Model file for the job. Use its own axes, mm. Face numbers are marked on the shaded views. A direction names the side the tool comes from. Round coordinates to 2 decimals unless told otherwise and drop trailing zeros. Order: outer loops, then holes, each group sorted by start corner. A loop starts at its lowest first (then second) coordinate and runs counter-clockwise, first axis right, second up. Notation, with made-up numbers: (85, 19.5) - (124, 19.5) arc R24 cw to (124, 45.5) - close; hole circle Ø10 at (49.5, 61.25). An arc over 180 degrees is marked (long way). Answer as CSV lines item,"result". Start each with the question number.
1. Band-saw the part on B-B on z = 21.75. List the corners of the cut face in (x, y) (3 decimals).
2. Wall check: line 1 along Y through (x, z) = (0, 26.65); line 2 along X through (y, z) = (13.5, 34); line 3 along Y through (x, z) = (20, 31.75). Give the ranges that are in metal, low to high. Write a range as [from, to].
3. Band-saw the part on A-A on y = 0. List the corners of the cut face in (x, z) (3 decimals).
4. Pin check, flat tips, straight feed: pin 1 Ø2.5 at (y, z) = (23.5, 32.5) entering from -X; pin 2 Ø4 at (x, y) = (3, -18.5) entering from +Z; pin 3 Ø6 at (x, z) = (4, 26) entering from +Y; pin 4 Ø8 at (x, z) = (40.5, 25) entering from +Y. Stop position of each tip, or through.
5. Band-saw the part on D-D on x = 52.5. List the corners of the cut face in (y, z).
6. Band-saw the part on C-C on x = 0. State how many separate pieces and enclosed holes the cut face has, then the cut area to 3 significant figures.
7. 3-axis set-ups, long thin cutter, end or side, ignore diameter. For the marked faces 1, 2, 3 and 4: which of +Z, -Z, +X, -X, +Y, -Y reach the whole face in a straight line?
8. Pull direction Y, two halves, no side cores. Call the marked faces 5, 6, 7 and 8: released by +Y, released by -Y, zero draft, split by the parting line, or undercut.
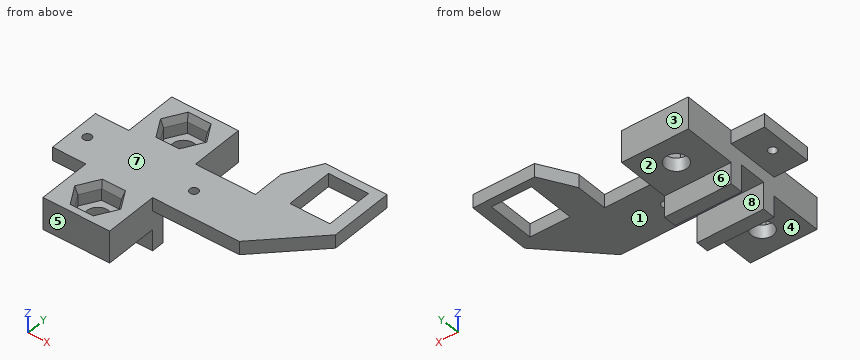
```python
from build123d import *

# Parameters (mm, degrees)
SKETCH2_W                = 25
SKETCH2_H                = 20
BOSS_EXTRUDE1_DEPTH      = 30
SKETCH3_W                = 20.25
SKETCH3_H                = 10.25
CUT_EXTRUDE1_DEPTH       = 26
SKETCH4_W                = 50
SKETCH4_H                = 20
BOSS_EXTRUDE2_DEPTH      = 5
SKETCH6_R                = 1.6
CUT_EXTRUDE2_DEPTH       = 36
SKETCH9_W                = 5
SKETCH9_H                = 20
BOSS_EXTRUDE3_DEPTH      = 40
BOSS_EXTRUDE5_START      = -5
SKETCH14_W               = 30
SKETCH14_H               = 24
BOSS_EXTRUDE5_DEPTH      = 5
SKETCH19_W               = 15
SKETCH19_H               = 18
CUT_EXTRUDE5_DEPTH       = 36
CHAMFER1_SIZE            = 12
CHAMFER1_SIZE2           = 6.92820323
CHAMFER2_SIZE            = 20
SKETCH20_W               = 25
SKETCH20_H               = 9
BOSS_EXTRUDE6_DEPTH      = 20
BOSS_EXTRUDE6_DEPTH_BACK = 40
SKETCH21_W               = 25
SKETCH21_H               = 20
CUT_EXTRUDE6_DEPTH       = 15
CUT_EXTRUDE7_DEPTH       = 7
SKETCH23_W               = 25
SKETCH23_H               = 20
BOSS_EXTRUDE7_DEPTH      = 3
SKETCH24_R               = 4.15
CUT_EXTRUDE8_DEPTH       = 14
CHAMFER3_SIZE            = 1
CHAMFER3_SIZE2           = 2.747477419


with BuildPart() as part:
    # Sketch2 → Boss-Extrude1 (new body)
    with BuildSketch(Plane.XY):
        Rectangle(SKETCH2_W, SKETCH2_H)
    extrude(amount=BOSS_EXTRUDE1_DEPTH)

    # Sketch3 → Cut-Extrude1 (cut, through all)
    with BuildSketch(Plane.ZY.offset(12.5)):
        with Locations((15, 0)):
            Rectangle(SKETCH3_W, SKETCH3_H)
    extrude(amount=-CUT_EXTRUDE1_DEPTH, mode=Mode.SUBTRACT)

    # Sketch4 → Boss-Extrude2 (add)
    with BuildSketch(Plane.XY.offset(30)):
        Rectangle(SKETCH4_W, SKETCH4_H)
    extrude(amount=BOSS_EXTRUDE2_DEPTH)

    # Sketch6 → Cut-Extrude2 (cut, through all)
    with BuildSketch(Plane.XY.offset(35)):
        with Locations((-20, 0)):
            Circle(SKETCH6_R)
        with Locations((20, 0)):
            Circle(SKETCH6_R)
    extrude(amount=-CUT_EXTRUDE2_DEPTH, mode=Mode.SUBTRACT)

    # Sketch9 → Boss-Extrude3 (add)
    with BuildSketch(Plane(origin=(25, 0, 0), x_dir=(0, 0, -1), z_dir=(1, 0, 0))):
        with Locations((-32.5, 0)):
            Rectangle(SKETCH9_W, SKETCH9_H)
    extrude(amount=BOSS_EXTRUDE3_DEPTH)

    # Sketch14 → Boss-Extrude5 (add)
    with BuildSketch(Plane.XY.offset(35).offset(BOSS_EXTRUDE5_START)):
        with Locations((50, 22)):
            Rectangle(SKETCH14_W, SKETCH14_H)
    extrude(amount=BOSS_EXTRUDE5_DEPTH)

    # Sketch19 → Cut-Extrude5 (cut, through all)
    with BuildSketch(Plane.XY.offset(35)):
        with Locations((53, 22)):
            Rectangle(SKETCH19_W, SKETCH19_H)
    extrude(amount=-CUT_EXTRUDE5_DEPTH, mode=Mode.SUBTRACT)

    # Chamfer1
    chamfer1_edges = [part.edges().sort_by_distance(p)[0] for p in [
        (35, 34, 32.5),
    ]]
    chamfer1_side = [part.faces().sort_by_distance(p)[0] for p in [
        (35, 22, 32.5),
    ]]
    chamfer(chamfer1_edges, length=CHAMFER1_SIZE, length2=CHAMFER1_SIZE2, reference=chamfer1_side[0])

    # Chamfer2
    chamfer2_edges = [part.edges().sort_by_distance(p)[0] for p in [
        (65, -10, 32.5),
    ]]
    chamfer(chamfer2_edges, length=CHAMFER2_SIZE)

    # Sketch20 → Boss-Extrude6 (add, two sides)
    with BuildSketch(Plane(origin=(0, 10, 0), x_dir=(1, 0, 0), z_dir=(0, 1, 0))) as boss_extrude6_sk:
        with Locations((0, -30.5)):
            Rectangle(SKETCH20_W, SKETCH20_H)
    extrude(amount=BOSS_EXTRUDE6_DEPTH)
    extrude(boss_extrude6_sk.sketch, amount=-BOSS_EXTRUDE6_DEPTH_BACK)

    # Sketch21 → Cut-Extrude6 (cut)
    with BuildSketch(Plane(origin=(0, 0, 0), x_dir=(-1, 0, 0), z_dir=(0, 0, -1))):
        Rectangle(SKETCH21_W, SKETCH21_H)
    extrude(amount=-CUT_EXTRUDE6_DEPTH, mode=Mode.SUBTRACT)

    # Sketch22 → Cut-Extrude7 (cut)
    with BuildSketch(Plane.XY.offset(35)):
        Polygon((7.5, 20), (3.75, 26.495190528), (-3.75, 26.495190528), (-7.5, 20), (-3.75, 13.504809472), (3.75, 13.504809472), align=None)
        Polygon((7.5, -20), (3.75, -13.504809472), (-3.75, -13.504809472), (-7.5, -20), (-3.75, -26.495190528), (3.75, -26.495190528), align=None)
    extrude(amount=-CUT_EXTRUDE7_DEPTH, mode=Mode.SUBTRACT)

    # Sketch23 → Boss-Extrude7 (add)
    with BuildSketch(Plane(origin=(0, 0, 26), x_dir=(-1, 0, 0), z_dir=(0, 0, -1))):
        with Locations((0, 20)):
            Rectangle(SKETCH23_W, SKETCH23_H)
        with Locations((0, -20)):
            Rectangle(SKETCH23_W, SKETCH23_H)
    extrude(amount=BOSS_EXTRUDE7_DEPTH)

    # Sketch24 → Cut-Extrude8 (cut, through all)
    with BuildSketch(Plane.XY.offset(28)):
        with Locations((0, 20)):
            Circle(SKETCH24_R)
        with Locations((0, -20)):
            Circle(SKETCH24_R)
    extrude(amount=-CUT_EXTRUDE8_DEPTH, mode=Mode.SUBTRACT)

    # Chamfer3
    chamfer3_edges = [part.edges().sort_by_distance(p)[0] for p in [
        (5.625, 16.752404736, 35),
        (5.625, 23.247595264, 35),
        (0, 26.495190528, 35),
        (-5.625, 23.247595264, 35),
        (-5.625, 16.752404736, 35),
        (0, 13.504809472, 35),
        (5.625, -23.247595264, 35),
        (5.625, -16.752404736, 35),
        (0, -13.504809472, 35),
        (-5.625, -16.752404736, 35),
        (-5.625, -23.247595264, 35),
        (0, -26.495190528, 35),
    ]]
    chamfer3_side = [part.faces().sort_by_distance(p)[0] for p in [
        (16.470883445, 3.451620449, 35),
    ]]
    chamfer(chamfer3_edges, length=CHAMFER3_SIZE, length2=CHAMFER3_SIZE2, reference=chamfer3_side[0])


solid = part.part
```
Reply:
1,outline,"(-12.5, -10) - (12.5, -10) - (12.5, -5.125) - (-12.5, -5.125) - close; (-12.5, 5.125) - (12.5, 5.125) - (12.5, 10) - (-12.5, 10) - close"
2,line 1,"y = [-30, -24.15], [-15.85, 15.85], [24.15, 30]"
2,line 2,"x = [-12.5, -4.48], [4.48, 12.5], [35, 45.5], [60.5, 65]"
2,line 3,"y = [-10, -1.6], [1.6, 10]"
3,outline,"(-25, 30) - (-21.6, 30) - (-21.6, 35) - (-25, 35) - close; (-18.4, 30) - (-12.5, 30) - (-12.5, 25.125) - (12.5, 25.125) - (12.5, 30) - (18.4, 30) - (18.4, 35) - (-18.4, 35) - close; (21.6, 30) - (55, 30) - (55, 35) - (21.6, 35) - close"
4,pin 1,"stops at x = -12.5"
4,pin 2,"stops at z = 28"
4,pin 3,"stops at y = 30"
4,pin 4,"passes through"
5,outline,"(-2.5, 30) - (13, 30) - (13, 35) - (-2.5, 35) - close; (31, 30) - (34, 30) - (34, 35) - (31, 35) - close"
6,separate pieces,"3"
6,enclosed holes,"0"
6,area,"506 mm2"
7,face 1,"-Z, +X, +Y, -Y"
7,face 2,"-Z, +X, -X, +Y"
7,face 3,"+Z, -Z, -X, +Y"
7,face 4,"-Z, +X, -X, -Y"
8,face 5,"released by -Y"
8,face 6,"released by +Y"
8,face 7,"zero draft"
8,face 8,"undercut"
